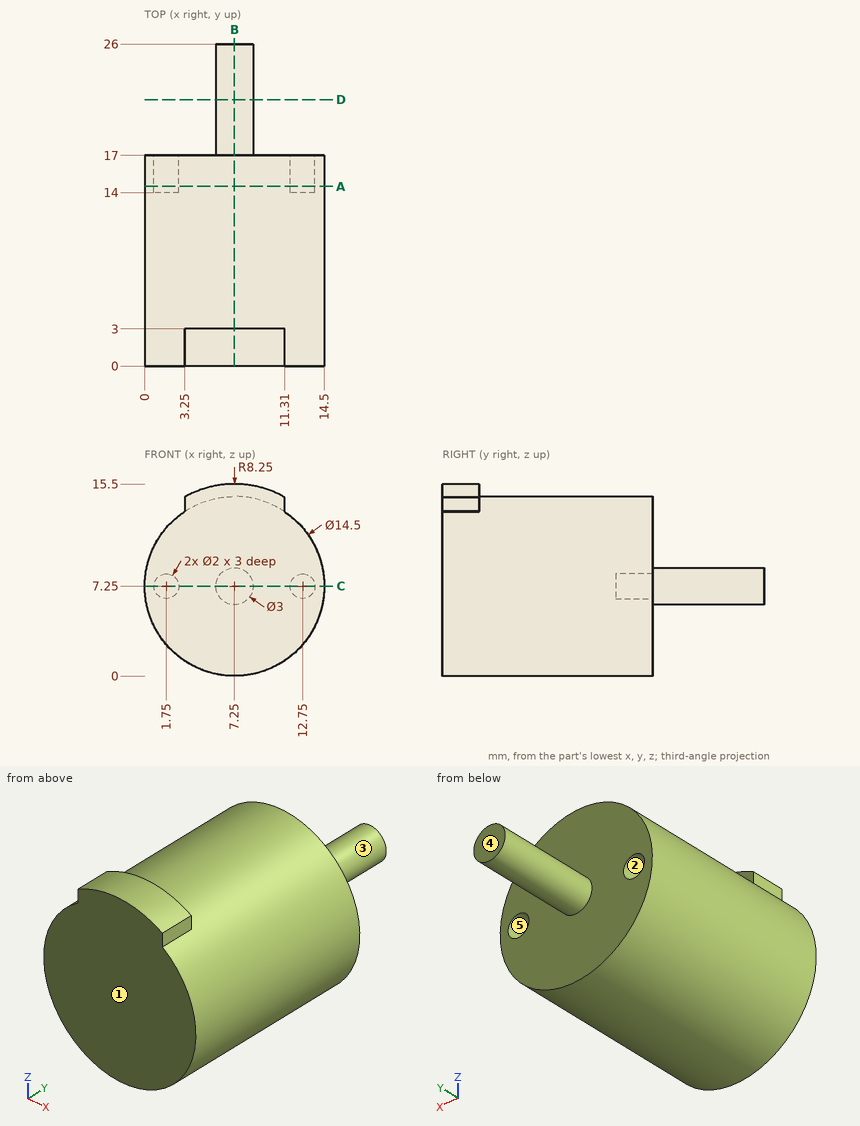
Job drawing, mm, ordinate dimensions from the low corner. One solid piece. A direction names the side the tool comes from. Round coordinates to 2 decimals unless told otherwise and drop trailing zeros. Loops run counter-clockwise (first coordinate to the right, second up) from the corner with the lowest first, then second, coordinate; pieces in that order, holes last. Notation, with made-up numbers: M 43,9 L 94,9 A20 ccw 94,27 Z; hole C 74.25,-28.75 d8. An arc over 180 degrees is marked long. One line per question, with ' | ' between items. Start each with the question number.
Item 1: Which spindle directions (+Z, -Z, +X, -X, +Y, -Y) get a long thin tool onto all of the face, cutting with end or side? Do the marked faces 1 and 2. Say none if no direction does.
Item 2: Two-plate mould, pull along X, no slides. Class the marked faces 3, 4 and 5: pulls with the +X half, pulls with the -X half, needs draft (parallel to the pull), parting line crosses it, or undercut.
Item 3: Wall check: line 1 (X direction, y = 16.1, z = 7.25); line 2 (Y direction, x = 5, z = 13.25); line 3 (Y direction, x = 10.5, z = 14.5). Give the ranges that are in metal, low to high.
Item 4: Pin check, flat tips, straight feed: pin 1 Ø1 at (x, z) = (1.5, 7.5) entering from +Y; pin 2 Ø1.6 at (x, z) = (12.5, 7.5) entering from +Y; pin 3 Ø1.3 at (y, z) = (2, 14) entering from -X. Stop position of each tip, or through.
Item 5: Cut at A-A, the plane y = 14.5. Write the cut outline in (x, z).
Item 6: Cut at B-B, the plane x = 7.25. Write the cut outline in (y, z).
Item 7: Cut at D-D, the plane y = 21.5. Write the cut outline in (x, z).
Item 8: Cut at C-C, the plane z = 7.25. Write the cut outline in (x, y).
Responses:
1) face 1: +Z, -Z, +X, -X, -Y | face 2: +Y
2) face 3: parting line crosses it | face 4: needs draft | face 5: undercut
3) line 1: x = 0 to 0.75, 2.75 to 11.75, 13.75 to 14.5 | line 2: y = 0 to 17 | line 3: y = 0 to 3
4) pin 1: stops at y = 14 | pin 2: stops at y = 17 | pin 3: stops at x = 3.25
5) outline: C 7.25,7.25 d14.5; hole C 1.75,7.25 d2; hole C 12.75,7.25 d2
6) outline: M 0,0 L 17,0 L 17,5.75 L 26,5.75 L 26,8.75 L 17,8.75 L 17,14.5 L 3,14.5 L 3,15.5 L 0,15.5 Z
7) outline: C 7.25,7.25 d3
8) outline: M 0,0 L 14.5,0 L 14.5,17 L 13.75,17 L 13.75,14 L 11.75,14 L 11.75,17 L 8.75,17 L 8.75,26 L 5.75,26 L 5.75,17 L 2.75,17 L 2.75,14 L 0.75,14 L 0.75,17 L 0,17 Z
